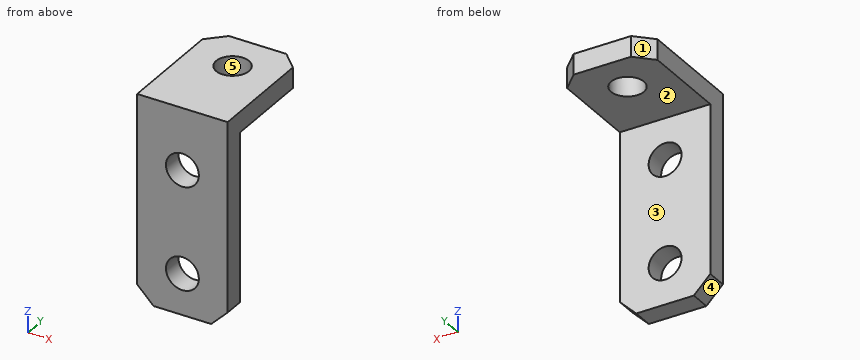
```python
from build123d import *

# Parameters (mm, degrees)
SKETCH_1_W      = 22
SKETCH_1_H      = 50
SKETCH_1_R      = 4
EXTRUDE_1_DEPTH = 5
SKETCH_2_W      = 22
SKETCH_2_H      = 25
SKETCH_2_R      = 4
EXTRUDE_2_DEPTH = 5
CHAMFER_1_SIZE  = 4


with BuildPart() as part:
    # 草图1 → 凸台-拉伸1 (new body)
    with BuildSketch(Plane(origin=(0, 0, 0), x_dir=(1, 0, 0), z_dir=(0, 1, 0))):
        with Locations((-2.015873016, -3.888888889)):
            Rectangle(SKETCH_1_W, SKETCH_1_H)
        with Locations(Location((-2.015873016, 11.111111111, 0), (0, 0, 270))):
            Circle(SKETCH_1_R, mode=Mode.SUBTRACT)
        with Locations(Location((-2.015873016, -13.888888889, 0), (0, 0, 270))):
            Circle(SKETCH_1_R, mode=Mode.SUBTRACT)
    extrude(amount=EXTRUDE_1_DEPTH)

    # 草图2 → 凸台-拉伸2 (add)
    with BuildSketch(Plane.XY.offset(28.888888889)):
        with Locations((-2.015873016, 17.5)):
            Rectangle(SKETCH_2_W, SKETCH_2_H)
        with Locations((-2.015873016, 20)):
            Circle(SKETCH_2_R, mode=Mode.SUBTRACT)
    extrude(amount=-EXTRUDE_2_DEPTH)

    # 倒角1
    chamfer_1_edges = [part.edges().sort_by_distance(p)[0] for p in [
        (-13.015873016, 30, 26.388888889),
        (8.984126984, 30, 26.388888889),
        (-13.015873016, 2.5, -21.111111111),
        (8.984126984, 2.5, -21.111111111),
    ]]
    chamfer(chamfer_1_edges, length=CHAMFER_1_SIZE)


solid = part.part
```
Source: CAD feature listing. Evaluate the final solid. Frame: model axes, mm. Face numbers are marked on the shaded views. A direction names the side the tool comes from. Round coordinates to 2 decimals unless told otherwise and drop trailing zeros. Order: outer loops, then holes, each group sorted by start corner. A loop starts at its lowest first (then second) coordinate and runs counter-clockwise, first axis right, second up. Notation, with made-up numbers: (74.5, -19) -> (112.5, -19) arc R25 cw to (112.5, 6) -> close; hole circle Ø6 at (9, 35.5). An arc over 180 degrees is marked (long way). One line per item, written item: value. Start each with the question number.
Q1. Material intervals for probe 1 along Y at (x, z) = (4.25, 11); probe 2 along Z at (x, y) = (-9.25, 24.75); probe 3 along X at (y, z) = (17.75, 27.5), sorted ascending.
Q2. Section query A-A (y = 20). Return the cut outline in (x, z).
Q3. Section query B-B (z = 24.5). Return the cut outline in (x, y).
Q4. Draft query along X for the marked faces 3, 4 and 5. Return one class per face: pulls with the +X half, pulls with the -X half, needs draft (parallel to the pull), parting line crosses it, or undercut.
Q5. Pin query (flat end, axial travel): pin 1 (9 mm diameter, centred on x = -2.02, z = 13.89, fed in from +Y); pin 2 (4 mm diameter, centred on x = -5, y = 10, fed in from -Z). Return the tip coordinate at first contact, or that it passes through.
Q6. Access query for the marked faces 1 and 2. Directions: +Z, -Z, +X, -X, +Y, -Y. A direction counts if a zero-diameter tool reaches every point of the face in a straight line with its end or side. Return the directions, or none.
Q7. Section query D-D (x = 3.5). Return the cut outline in (y, z).
Q8. Section query C-C (x = -4). Return the cut outline in (y, z).
Findings below:
1. probe 1: 0 to 5
1. probe 2: 23.89 to 28.89
1. probe 3: -13.02 to -5.32, 1.29 to 8.98
2. outline: (-13.02, 23.89) -> (-6.02, 23.89) -> (-6.02, 28.89) -> (-13.02, 28.89) -> close; (1.98, 23.89) -> (8.98, 23.89) -> (8.98, 28.89) -> (1.98, 28.89) -> close
3. outline: (-13.02, 0) -> (8.98, 0) -> (8.98, 26) -> (4.98, 30) -> (-9.02, 30) -> (-13.02, 26) -> close; hole circle Ø8 at (-2.02, 20)
4. face 3: needs draft
4. face 4: pulls with the -X half
4. face 5: undercut
5. pin 1: y = 5
5. pin 2: z = 23.89
6. face 1: +Z, -Z, -X, +Y
6. face 2: -Z, +X, -X, +Y
7. outline: (0, -21.11) -> (5, -21.11) -> (5, 23.89) -> (30, 23.89) -> (30, 28.89) -> (0, 28.89) -> close
8. outline: (0, -21.11) -> (5, -21.11) -> (5, -14.58) -> (0, -14.58) -> close; (0, -7.64) -> (5, -7.64) -> (5, 10.42) -> (0, 10.42) -> close; (0, 17.36) -> (5, 17.36) -> (5, 23.89) -> (16.53, 23.89) -> (16.53, 28.89) -> (0, 28.89) -> close; (23.47, 23.89) -> (30, 23.89) -> (30, 28.89) -> (23.47, 28.89) -> close
